Autodesk Inventor part; units mm, degrees
ref_plane "YZ Plane" through (0, 0, 0) normal (1, 0, 0) x (0, 1, 0)
ref_plane "XZ Plane" through (0, 0, 0) normal (0, 1, 0) x (-1, 0, 0)
ref_plane "XY Plane" through (0, 0, 0) normal (0, 0, 1) x (1, 0, 0)
sketch "スケッチ1" plane through (0, 0, 0) normal (0, 1, 0) x (-1, 0, 0)
  line L0 (0, 0) -> (16, 0)
  line L1 (16, 0) -> (16, -30)
  line L2 (16, -30) -> (0, -30)
  line L3 (0, -30) -> (0, 0)
  circle A0 centre (8, -3.5) radius 3.5
  circle A1 centre (8, -26.5) radius 3.5
  line L4 (16, -3.5) -> (0, -3.5)
  line L5 (16, -26.5) -> (-0.2656, -26.5)
  point P0 (8, 0)
  point P1 (11.5, -3.5)
  point P2 (4.5, -3.5)
  point P3 (0, -26.5)
  point P4 (4.5, -26.5)
  point P5 (11.5, -26.5)
  dimension "d0" = 16
  dimension "d1" = 30
  dimension "d2" = 7
extrude "押し出し1" add sketch "スケッチ1" along normal blind 1.5 contours A0 L4 | L4 A0 L1 L5 A1 L3 | A0 L4 | L5 A1 | A1 L5
properties part number "external_input"
Geometry check sheet. Reference: the model listing, model coordinates, mm. A direction names the side the tool comes from. Give positions to 0.01 mm unless a question says otherwise; leave off trailing zeros. Loops run counter-clockwise (first coordinate to the right, second up) from the corner with the lowest first, then second, coordinate; pieces in that order, holes last. Notation, with made-up numbers: (21.25, 80) -> (52.25, 80) arc R6 ccw to (52.25, 84) -> close; hole circle Ø10 at (-13, 39). An arc over 180 degrees is marked (long way). Answer in a Markdown table with one row per item. Add a question column.
1) Cross-section at A-A on y = 0.65. Record the boundary of the cut face in (x, z), and give its area (3 significant figures).
2) Set-up check for faces 1 (the face through (-2, 1, -26.5)), 2 (the face through (-14, 1, -26.5)), 3 (the face through (-2, 1, -3.5)): record each of +Z, -Z, +X, -X, +Y, -Y from which the full face is reachable in a straight line by a thin tool's end or side.
3) Material ranges on probe 1 along Z at (x, y) = (-15, 0.8); probe 2 along X at (y, z) = (0.3, -28.25); probe 3 along Z at (x, y) = (-9, 1.1), recorded low to high. Write a range as from..to.
4) Cross-section at B-B on x = -13.75. Record the boundary of the cut face in (y, z), and give its area (3 significant figures).
5) Gauge pin test, flat end, axial feed: P1, Ø0.8, axis at x = -3, y = 0.5, coming from the +Z side. Record the tip position at first contact, or that the pin passes through.
Outcome:
| question | item | result |
|---|---|---|
| 1 | outline | (-16, -26.5) -> (-11.5, -26.5) arc R3.5 ccw to (-4.5, -26.5) -> (0, -26.5) -> (0, -3.5) -> (-4.5, -3.5) arc R3.5 ccw to (-11.5, -3.5) -> (-16, -3.5) -> close |
| 1 | area | 406 mm^2 |
| 2 | face 1 | -Z, +X, +Y, -Y |
| 2 | face 2 | -Z, -X, +Y, -Y |
| 2 | face 3 | +Z, +X, +Y, -Y |
| 3 | probe 1 | z = -26.5..-3.5 |
| 3 | probe 2 | x = -11.03..-4.97 |
| 3 | probe 3 | z = -29.85..-0.15 |
| 4 | outline | (0, -26.5) -> (1.5, -26.5) -> (1.5, -3.5) -> (0, -3.5) -> close |
| 4 | area | 34.5 mm^2 |
| 5 | P1 | stops at z = -3.5 |
